The listing builds one solid part. Answer for the finished solid, in the listing's coordinates (mm). A direction names the side the tool comes from. Give positions to 0.01 mm unless a question says otherwise; leave off trailing zeros. Use a Markdown table: item, result. Add a question column.
1) Straight lines are drawn through the part: line 1 (X direction, y = 24.5, z = 5); line 2 (Y direction, x = 25.5, z = 7.5); line 3 (X direction, y = 36, z = 4.5). For each, find the intervals that lie inside material, in ascending order.
2) For faces 1 (the face through (80.326, 33.452, 9.108)), 2 (the face through (42, 0, 4)), 3 (the face through (-1.4, 18.52, 8.93)), 4 (the face through (28, 35, 3.5)), 5 (the face through (45, 36.5, 3)), determine the directions among +Z, -Z, +X, -X, +Y, -Y from which every point of the face is accessible in a straight line to the end or side of a thin tool.
3) The mould has two halves that part along Y. Classify faces 6 (the face through (-2, 19, 4)), 7 (the face through (33.009, 34, 6)), 8 (the face through (86.4, 0.57, 3.7)): released by +Y, released by -Y, zero draft, split by the parting line, or undercut.
4) Flat-ended cylindrical pins translate along their axes: pin 1 (1 mm diameter, centred on x = 9.5, y = 17.5, fed in from -Z); pin 2 (0.6 mm diameter, centred on x = 28, y = 34.5, fed in from -Z); pin 3 (0.8 mm diameter, centred on x = 72.5, y = 37, fed in from +Z). Find the tip coordinate at first contact, or state that the pin passes through.
5) Find section D-D, the plane y = 5.4. State how many separate pieces and enclosed holes the cut face has, plus the area to 3 significant figures.
from build123d import *
from OCP.BRepAlgoAPI import BRepAlgoAPI_Cut
from OCP.TopTools import TopTools_ListOfShape

# Parameters (mm, degrees)
EXTRUDE_1_DEPTH      = 9.5
CUT_EXTRUDE_1_DEPTH  = 8.5
SKETCH_4_R           = 2.5
SKETCH_4_W           = 10
SKETCH_4_H           = 2
SKETCH_4_W_2         = 5
EXTRUDE_2_DEPTH      = 5
SKETCH_10_W          = 8.8
SKETCH_10_H          = 6
CUT_EXTRUDE_3_DEPTH  = 2
CUT_EXTRUDE_4_DEPTH  = 3
FILLET_4_R           = 2
FILLET_5_R           = 2
SKETCH_5_R           = 0.8
CUT_EXTRUDE_5_DEPTH  = 10
SKETCH_7_R           = 0.8
CUT_EXTRUDE_6_DEPTH  = 10
SKETCH_6_R           = 0.8
CUT_EXTRUDE_7_DEPTH  = 10
SKETCH_8_R           = 0.8
CUT_EXTRUDE_8_DEPTH  = 10
SKETCH_12_R          = 2
CUT_EXTRUDE_9_DEPTH  = 1
SKETCH_14_W          = 1.5
SKETCH_14_H          = 5
CUT_EXTRUDE_11_DEPTH = 1
SKETCH_15_W          = 1.5
SKETCH_15_H          = 5
CUT_EXTRUDE_12_DEPTH = 1
SKETCH_16_W          = 1.5
SKETCH_16_H          = 5
CUT_EXTRUDE_13_DEPTH = 1
SKETCH_18_W          = 3
SKETCH_18_H          = 3
SKETCH_18_W_2        = 4
SKETCH_18_H_2        = 13.499999703
EXTRUDE_3_DEPTH      = 5
SKETCH_20_W          = 11.8
SKETCH_20_H          = 1.5
CUT_EXTRUDE_16_DEPTH = 1
EXTRUDE_START        = 0.2
SKETCH_21_W          = 85
SKETCH_21_H          = 33.499999703
SKETCH_21_R          = 2
EXTRUDE_4_DEPTH      = 0.2
CUT_EXTRUDE_17_DEPTH = 1
SKETCH_22_W          = 7.8
SKETCH_22_H          = 1
CUT_EXTRUDE_18_DEPTH = 1


with BuildPart() as part:
    # 草图2 → 凸台-拉伸1 (new body)
    with BuildSketch(Plane.XY):
        with BuildLine():
            Line((0, 0), (85, 0))
            ThreePointArc((85, 0), (86.414213562, 0.585786438), (87, 2))
            Line((87, 2), (87, 35.5))
            ThreePointArc((87, 35.5), (86.41421356, 36.914213565), (84.999999993, 37.5))
            Line((84.999999993, 37.5), (-7e-09, 37.499999703))
            ThreePointArc((-7e-09, 37.499999703), (-1.414213565, 36.914213263), (-2, 35.499999703))
            Line((-2, 35.499999703), (-2, 1.999999703))
            ThreePointArc((-2, 1.999999703), (-1.414213353, 0.585786351), (0, 0))
        make_face()
    extrude(amount=EXTRUDE_1_DEPTH)

    # 草图3 → 切除-拉伸1 (cut)
    with BuildSketch(Plane(origin=(0, 0, 0), x_dir=(-1, 0, 0), z_dir=(0, 0, -1))):
        with BuildLine():
            Line((-83, 2), (-2.008987521, 2))
            ThreePointArc((-2.008987521, 2), (-0.594773959, 2.585786438), (-0.008987521, 4))
            Line((-0.008987521, 4), (-0.008987521, 33.499999703))
            ThreePointArc((-0.008987521, 33.499999703), (-0.594773959, 34.914213266), (-2.008987521, 35.499999703))
            Line((-2.008987521, 35.499999703), (-83, 35.499999703))
            ThreePointArc((-83, 35.499999703), (-84.414213562, 34.914213266), (-85, 33.499999703))
            Line((-85, 33.499999703), (-85, 4))
            ThreePointArc((-85, 4), (-84.414213562, 2.585786438), (-83, 2))
        make_face()
    extrude(amount=-CUT_EXTRUDE_1_DEPTH, mode=Mode.SUBTRACT)

    # 草图4 → 凸台-拉伸2 (add)
    with BuildSketch(Plane(origin=(0, 0, 8.5), x_dir=(-1, 0, 0), z_dir=(0, 0, -1))):
        with Locations((-81.8, 32.099999703)):
            Circle(SKETCH_4_R)
        with Locations((-8.008987521, 32.099999703)):
            Circle(SKETCH_4_R)
        with Locations((-8.008987521, 5.4)):
            Circle(SKETCH_4_R)
        with Locations((-81.8, 5.4)):
            Circle(SKETCH_4_R)
        with Locations((-28.008987521, 34.499999703)):
            Rectangle(SKETCH_4_W, SKETCH_4_H)
        with Locations((-62.5, 3)):
            Rectangle(SKETCH_4_W_2, SKETCH_4_H)
    extrude(amount=EXTRUDE_2_DEPTH)

    # 草图10 → 切除-拉伸3 (cut)
    with BuildSketch(Plane(origin=(-1.31e-07, 37.499999703, 0), x_dir=(1.0, 3.4902577560140295e-09, 0), z_dir=(-3.4902577560140295e-09, 1.0, 0))):
        with Locations((45.500000124, -6.5)):
            Rectangle(SKETCH_10_W, SKETCH_10_H)
        with Locations((70.800000124, -6.5)):
            Rectangle(SKETCH_10_W, SKETCH_10_H)
    extrude(amount=-CUT_EXTRUDE_3_DEPTH, mode=Mode.SUBTRACT)

    # 草图11 → 切除-拉伸4 (cut)
    with BuildSketch(Plane.ZY.offset(2)):
        with BuildLine():
            Line((0, 20.349999703), (0, 17.149999703))
            ThreePointArc((0, 17.149999703), (1.6, 18.749999703), (0, 20.349999703))
        make_face()
    extrude(amount=-CUT_EXTRUDE_4_DEPTH, mode=Mode.SUBTRACT)

    # 圆角4
    fillet_4_edges = [part.edges().sort_by_distance(p)[0] for p in [
        (80.099999993, 37.499999983, 9.5),
        (86.41421356, 36.914213565, 9.5),
        (87, 18.75, 9.5),
        (86.414213562, 0.585786438, 9.5),
        (42.5, 0, 9.5),
        (-1.414213396, 0.585786394, 9.5),
        (-2, 18.749999703, 9.5),
        (-1.414213565, 36.914213263, 9.5),
        (20.549999993, 37.499999775, 9.5),
    ]]
    fillet(fillet_4_edges, radius=FILLET_4_R - 0.0001)  # a hair under: the kernel refuses the full size

    # 圆角5
    fillet_5_edges = [part.edges().sort_by_distance(p)[0] for p in [
        (58.149999993, 37.499999906, 9.5),
    ]]
    fillet(fillet_5_edges, radius=FILLET_5_R)

    # 草图5 → 切除-拉伸5 (cut)
    with BuildSketch(Plane(origin=(0, 0, 3.5), x_dir=(-1, 0, 0), z_dir=(0, 0, -1))):
        with Locations((-81.8, 32.099999703)):
            Circle(SKETCH_5_R)
    extrude(amount=-CUT_EXTRUDE_5_DEPTH, mode=Mode.SUBTRACT)

    # 草图7 → 切除-拉伸6 (cut)
    with BuildSketch(Plane(origin=(0, 0, 3.5), x_dir=(-1, 0, 0), z_dir=(0, 0, -1))):
        with Locations((-8.008987521, 5.4)):
            Circle(SKETCH_7_R)
    extrude(amount=-CUT_EXTRUDE_6_DEPTH, mode=Mode.SUBTRACT)

    # 草图6 → 切除-拉伸7 (cut)
    with BuildSketch(Plane(origin=(0, 0, 3.5), x_dir=(-1, 0, 0), z_dir=(0, 0, -1))):
        with Locations((-8.008987521, 32.099999703)):
            Circle(SKETCH_6_R)
    extrude(amount=-CUT_EXTRUDE_7_DEPTH, mode=Mode.SUBTRACT)

    # 草图8 → 切除-拉伸8 (cut)
    with BuildSketch(Plane(origin=(0, 0, 3.5), x_dir=(-1, 0, 0), z_dir=(0, 0, -1))):
        with Locations((-81.8, 5.4)):
            Circle(SKETCH_8_R)
    extrude(amount=-CUT_EXTRUDE_8_DEPTH, mode=Mode.SUBTRACT)

    # 草图12 → 切除-拉伸9 (cut)
    with BuildSketch(Plane.XY.offset(9.5)):
        with Locations((8.008987521, 32.099999703)):
            Circle(SKETCH_12_R)
        with Locations((81.8, 32.099999703)):
            Circle(SKETCH_12_R)
        with Locations((81.8, 5.4)):
            Circle(SKETCH_12_R)
        with Locations((8.008987521, 5.4)):
            Circle(SKETCH_12_R)
    extrude(amount=-CUT_EXTRUDE_9_DEPTH, mode=Mode.SUBTRACT)

    # 草图14 → 切除-拉伸11 (cut)
    with BuildSketch(Plane.XZ.offset(-35.499999703)):
        with Locations((50.65, 6)):
            Rectangle(SKETCH_14_W, SKETCH_14_H)
        with Locations((65.65, 6)):
            Rectangle(SKETCH_14_W, SKETCH_14_H)
    extrude(amount=-CUT_EXTRUDE_11_DEPTH, mode=Mode.SUBTRACT)

    # 草图15 → 切除-拉伸12 (cut)
    with BuildSketch(Plane.XZ.offset(-35.499999703)):
        with Locations((75.95, 6)):
            Rectangle(SKETCH_15_W, SKETCH_15_H)
    extrude(amount=-CUT_EXTRUDE_12_DEPTH, mode=Mode.SUBTRACT)

    # 草图16 → 切除-拉伸13 (cut)
    with BuildSketch(Plane.XZ.offset(-35.499999703)):
        with Locations((40.35, 6)):
            Rectangle(SKETCH_16_W, SKETCH_16_H)
    extrude(amount=-CUT_EXTRUDE_13_DEPTH, mode=Mode.SUBTRACT)

    # 草图18 → 凸台-拉伸3 (add)
    with BuildSketch(Plane(origin=(0, 0, 8.5), x_dir=(-1, 0, 0), z_dir=(0, 0, -1))):
        with Locations((-78.5, 9.5)):
            Rectangle(SKETCH_18_W, SKETCH_18_H)
        with Locations((-78.5, 27.999999703)):
            Rectangle(SKETCH_18_W, SKETCH_18_H)
        with Locations((-35.008987521, 18.749999852)):
            Rectangle(SKETCH_18_W_2, SKETCH_18_H_2)
    extrude(amount=EXTRUDE_3_DEPTH)

    # 草图20 → 切除-拉伸16 (cut)
    with BuildSketch(Plane.XZ.offset(-35.499999703)):
        with Locations((45.5, 2.75)):
            Rectangle(SKETCH_20_W, SKETCH_20_H)
        with Locations((70.8, 2.75)):
            Rectangle(SKETCH_20_W, SKETCH_20_H)
    extrude(amount=-CUT_EXTRUDE_16_DEPTH, mode=Mode.SUBTRACT)

    # 草图21 → 凸台-拉伸4 (add)
    with BuildSketch(Plane.XY.offset(9.5).offset(EXTRUDE_START)):
        with Locations((42.5, 18.749999852)):
            Rectangle(SKETCH_21_W, SKETCH_21_H)
        with Locations((8.008987521, 32.099999703)):
            Circle(SKETCH_21_R, mode=Mode.SUBTRACT)
        with Locations((8.008987521, 5.4)):
            Circle(SKETCH_21_R, mode=Mode.SUBTRACT)
        with Locations((81.8, 32.099999703)):
            Circle(SKETCH_21_R, mode=Mode.SUBTRACT)
        with Locations((81.8, 5.4)):
            Circle(SKETCH_21_R, mode=Mode.SUBTRACT)
    extrude(amount=-EXTRUDE_4_DEPTH)


with BuildPart() as cut_extrude_17_tool:
    # 草图19 → 切除-拉伸17 (new body)
    with BuildSketch(Plane(origin=(0, 0, 0), x_dir=(-1, 0, 0), z_dir=(0, 0, -1))):
        with BuildLine():
            Line((-84, 36.499999703), (-1.008987521, 36.499999703))
            ThreePointArc((-1.008987521, 36.499999703), (0.369417354, 35.949137378), (0.988510914, 34.599999703))
            Line((0.988510914, 34.599999703), (0.995506239, 20.349999703))
            Line((0.995506239, 20.349999703), (-0.008987521, 20.349999703))
            Line((-0.008987521, 20.349999703), (-0.008987521, 33.599999703))
            ThreePointArc((-0.008987521, 33.599999703), (-0.628081081, 34.949137378), (-2.006485957, 35.499999703))
            Line((-2.006485957, 35.499999703), (-83, 35.499999703))
            ThreePointArc((-83, 35.499999703), (-84.414213562, 34.914213266), (-85, 33.499999703))
            Line((-85, 33.499999703), (-85, 4))
            ThreePointArc((-85, 4), (-84.414213562, 2.585786438), (-83, 2))
            Line((-83, 2), (-2.006485957, 2))
            ThreePointArc((-2.006485957, 2), (-0.628081081, 2.550862325), (-0.008987521, 3.9))
            Line((-0.008987521, 3.9), (-0.008987521, 17.149999703))
            Line((-0.008987521, 17.149999703), (0.995506239, 17.149999703))
            Line((0.995506239, 17.149999703), (0.988510914, 2.9))
            ThreePointArc((0.988510914, 2.9), (0.369417354, 1.550862325), (-1.008987521, 1))
            Line((-1.008987521, 1), (-84, 1))
            ThreePointArc((-84, 1), (-85.414213562, 1.585786438), (-86, 3))
            Line((-86, 3), (-86, 34.499999703))
            ThreePointArc((-86, 34.499999703), (-85.414213562, 35.914213266), (-84, 36.499999703))
        make_face()
    extrude(amount=-CUT_EXTRUDE_17_DEPTH)


with BuildPart() as part_1:
    add(part.part)

    # 切除-拉伸17: cut by cut_extrude_17_tool, with a tolerance
    cut_extrude_17_stock = TopTools_ListOfShape()
    cut_extrude_17_stock.Append(part_1.part.wrapped)
    cut_extrude_17_tools = TopTools_ListOfShape()
    cut_extrude_17_tools.Append(cut_extrude_17_tool.part.wrapped)
    cut_extrude_17_cut = BRepAlgoAPI_Cut()
    cut_extrude_17_cut.SetArguments(cut_extrude_17_stock)
    cut_extrude_17_cut.SetTools(cut_extrude_17_tools)
    cut_extrude_17_cut.SetFuzzyValue(0.00001)
    cut_extrude_17_cut.Build()
    add(Compound.cast(cut_extrude_17_cut.Shape()).solids(), mode=Mode.REPLACE)

    # 草图22 → 切除-拉伸18 (cut)
    with BuildSketch(Plane(origin=(0, 0, 1), x_dir=(-1, 0, 0), z_dir=(0, 0, -1))):
        with Locations((-21.6, 1.5)):
            Rectangle(SKETCH_22_W, SKETCH_22_H)
    extrude(amount=-CUT_EXTRUDE_18_DEPTH, mode=Mode.SUBTRACT)


solid = part_1.part
The answers:
| question | item | result |
|---|---|---|
| 1 | line 1 | -2 to 0.01, 33.01 to 37.01, 85 to 87 |
| 1 | line 2 | 0 to 2, 33.5 to 37.5 |
| 1 | line 3 | -1.94 to 39.6, 51.4 to 64.9, 76.7 to 86.94 |
| 2 | face 1 | +Z |
| 2 | face 2 | +Z, -Z, +X, -X, -Y |
| 2 | face 3 | +Z, -X, +Y, -Y |
| 2 | face 4 | -Z |
| 2 | face 5 | none |
| 3 | face 6 | zero draft |
| 3 | face 7 | undercut |
| 3 | face 8 | released by -Y |
| 4 | pin 1 | z = 8.5 |
| 4 | pin 2 | z = 3.5 |
| 4 | pin 3 | z = 3.5 |
| 5 | separate pieces | 3 |
| 5 | enclosed holes | 0 |
| 5 | area | 161 mm2 |
